from build123d import *

# Parameters (mm, degrees)
SKETCH1_W           = 42
SKETCH1_H           = 42
BOSS_EXTRUDE1_DEPTH = 4
SKETCH2_W           = 10
SKETCH2_H           = 42
BOSS_EXTRUDE2_DEPTH = 11
SKETCH3_R           = 11
CUT_EXTRUDE1_DEPTH  = 11
FILLET1_R           = 3
SKETCH4_R           = 1.75
CUT_EXTRUDE2_DEPTH  = 21
SKETCH6_R           = 3
SKETCH6_R_2         = 1.5
CUT_EXTRUDE3_DEPTH  = 21


with BuildPart() as part:
    # Sketch1 → Boss-Extrude1 (new body)
    with BuildSketch(Plane.XY):
        Rectangle(SKETCH1_W, SKETCH1_H)
    extrude(amount=BOSS_EXTRUDE1_DEPTH)

    # Sketch2 → Boss-Extrude2 (add)
    with BuildSketch(Plane.XY.offset(4)):
        with Locations((-16, 0)):
            Rectangle(SKETCH2_W, SKETCH2_H)
    extrude(amount=BOSS_EXTRUDE2_DEPTH)

    # Sketch3 → Cut-Extrude1 (cut)
    with BuildSketch(Plane.XY.offset(4)):
        Circle(SKETCH3_R)
    extrude(amount=-CUT_EXTRUDE1_DEPTH, mode=Mode.SUBTRACT)

    # Fillet1
    fillet1_edges = [part.edges().sort_by_distance(p)[0] for p in [
        (-11, -21, 9.5),
        (-11, 21, 9.5),
        (21, -21, 2),
        (-21, -21, 7.5),
        (-21, 21, 7.5),
        (21, 21, 2),
    ]]
    fillet(fillet1_edges, radius=FILLET1_R)

    # Sketch4 → Cut-Extrude2 (cut)
    with BuildSketch(Plane.XY.offset(15)):
        with Locations((-15.5, 15.5)):
            Circle(SKETCH4_R)
        with Locations((-15.5, -15.5)):
            Circle(SKETCH4_R)
        with Locations((15.5, 15.5)):
            Circle(SKETCH4_R)
        with Locations((15.5, -15.5)):
            Circle(SKETCH4_R)
    extrude(amount=-CUT_EXTRUDE2_DEPTH, mode=Mode.SUBTRACT)

    # Sketch6 → Cut-Extrude3 (cut)
    with BuildSketch(Plane.ZY.offset(21)):
        with Locations((9.5, 6)):
            Circle(SKETCH6_R)
        with Locations((9.5, -11)):
            Circle(SKETCH6_R_2)
    extrude(amount=-CUT_EXTRUDE3_DEPTH, mode=Mode.SUBTRACT)


solid = part.part
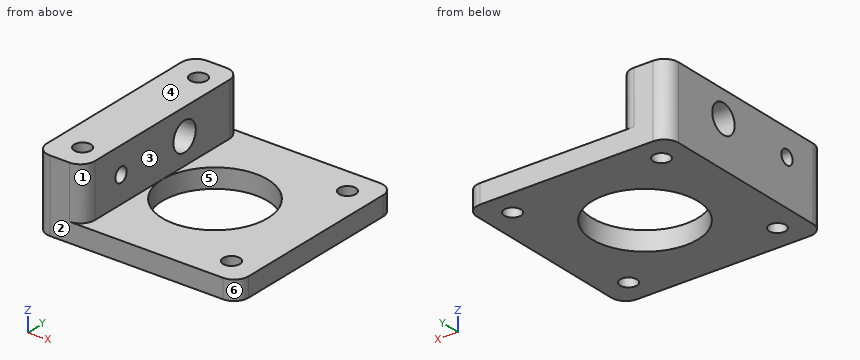
Work out the finished part from the listing and answer in its coordinate system (mm). Face numbers are marked on the shaded views. A direction names the side the tool comes from. Give positions to 0.01 mm unless a question says otherwise; leave off trailing zeros. Loops run counter-clockwise (first coordinate to the right, second up) from the corner with the lowest first, then second, coordinate; pieces in that order, holes last. Notation, with made-up numbers: (69, 47) - (123, 47) arc R13 ccw to (123, 59) - close; hole circle Ø8 at (58.25, 53.25). An arc over 180 degrees is marked (long way). Answer in a Markdown table with one row per item. Add a question column.
Q1. Consider line 1 along Y through (x, z) = (-18.25, 9.5); line 2 along Y through (x, z) = (-15.5, 4.25); line 3 along Y through (x, z) = (0, 2.95). Determine where each line is inside the solid, lowest interval first.
Q2. The part is cut by section C-C (y = 15.5). Determine the outline of the cut face in (x, z).
Q3. A tool of negligible diameter and unlimited length cuts with its end or side. For the marked faces 1, 2 and 3, from which of +Z, -Z, +X, -X, +Y, -Y can it reach the whole face along a straight path? Write none if from no direction.
Q4. Determine the mould class of the marked faces 4, 5 and 6 for opening direction Y: released by +Y, released by -Y, zero draft, split by the parting line, or undercut.
Q5. The part is cut by section A-A (z = 9.5). Determine the outline of the cut face in (x, y).
Q6. The part is cut by section B-B (x = 0). Determine the outline of the cut face in (y, z).
Q7. The part is cut by section D-D (x = 15.5). Determine the outline of the cut face in (y, z).
Q8. Each of these flat-tipped pins is pushed along its axis until it touches: P1, Ø2, axis at y = 6.5, z = 12.5, coming from the +X side; P2, Ø3, axis at x = 15.5, y = -15.5, coming from the -Z side; P3, Ø4, axis at x = 15.5, y = 15.5, coming from the +Z side. Where does it stop, or does it pass through?
Solution:
| question | item | result |
|---|---|---|
| 1 | line 1 | y = -20.99 to -12.5, -9.5 to 3, 9 to 20.99 |
| 1 | line 2 | y = -21 to -17.25, -13.75 to 13.75, 17.25 to 21 |
| 1 | line 3 | y = -21 to -11, 11 to 21 |
| 2 | outline | (-21, 0) - (-17.25, 0) - (-17.25, 15) - (-21, 15) - close; (-13.75, 0) - (13.75, 0) - (13.75, 4) - (-11, 4) - (-11, 15) - (-13.75, 15) - close; (17.25, 0) - (21, 0) - (21, 4) - (17.25, 4) - close |
| 3 | face 1 | +Z, +X, -Y |
| 3 | face 2 | +Z, -Z, +X, -X, -Y |
| 3 | face 3 | +Z, +X, +Y, -Y |
| 4 | face 4 | zero draft |
| 4 | face 5 | undercut |
| 4 | face 6 | released by -Y |
| 5 | outline | (-21, -18) arc R3 ccw to (-18, -21) - (-14, -21) arc R3 ccw to (-11, -18) - (-11, -12.5) - (-21, -12.5) - close; (-21, -9.5) - (-11, -9.5) - (-11, 3) - (-21, 3) - close; (-21, 9) - (-11, 9) - (-11, 18) arc R3 ccw to (-14, 21) - (-18, 21) arc R3 ccw to (-21, 18) - close; hole circle Ø3.5 at (-15.5, -15.5); hole circle Ø3.5 at (-15.5, 15.5) |
| 6 | outline | (-21, 0) - (-11, 0) - (-11, 4) - (-21, 4) - close; (11, 0) - (21, 0) - (21, 4) - (11, 4) - close |
| 7 | outline | (-21, 0) - (-17.25, 0) - (-17.25, 4) - (-21, 4) - close; (-13.75, 0) - (13.75, 0) - (13.75, 4) - (-13.75, 4) - close; (17.25, 0) - (21, 0) - (21, 4) - (17.25, 4) - close |
| 8 | P1 | stops at x = -11 |
| 8 | P2 | passes through |
| 8 | P3 | stops at z = 4 |
